Autodesk Inventor part; units mm, degrees
ref_plane "YZ Plane" through (0, 0, 0) normal (1, 0, 0) x (0, 1, 0)
ref_plane "XZ Plane" through (0, 0, 0) normal (0, 1, 0) x (-1, 0, 0)
ref_plane "XY Plane" through (0, 0, 0) normal (0, 0, 1) x (1, 0, 0)
sketch "Sketch1" plane through (0, 0, 0) normal (0, 1, 0) x (-1, 0, 0)
  circle A0 centre (0, 0) radius 3.9
  dimension "d0" = 7.8
extrude "Extrusion1" add sketch "Sketch1" along normal blind 5.2
sketch "Sketch2" plane through (0, 0, 0) normal (0, -1, 0) x (1, 0, 0)
  circle A0 centre (0, 0) radius 5.5
  dimension "d3" = 11
extrude "Extrusion2" add sketch "Sketch2" along normal blind 16.5
sketch "Sketch3" plane through (0, 5.2, 0) normal (0, 1, 0) x (1, 0, 0)
  circle A0 centre (0, 0) radius 2.9
  circle A1 centre (0, 0) radius 1
  dimension "d6" = 5.8
  dimension "d7" = 2
extrude "Extrusion3" cut sketch "Sketch3" against normal blind 10
fillet "Fillet1" radius 1 1 edges at (-1, 5.2, 0)
properties part number "Strom"
Part model, mm, in its own coordinate system. A direction names the side the tool comes from. Coordinates: 2 decimals unless noted, no trailing zeros. Order: outer loops, then holes, each group sorted by start corner. A loop starts at its lowest first (then second) coordinate and runs counter-clockwise, first axis right, second up. Notation, with made-up numbers: M 40.5,-17 L 67.5,-17 A6 cw 67.5,-11 Z; hole C 43,-31 d3. An arc over 180 degrees is marked long. One line per question, with ' | ' between items.
Q1. Drill centre lines: line 1 (Z direction, x = 0, y = 2); line 2 (Z direction, x = 0, y = -2); line 3 (X direction, y = 2.5, z = -0.5). Where is each one in solid material? Low to high.
A:
line 1: z = -3.9 to -2.9, -1 to 1, 2.9 to 3.9 | line 2: z = -5.5 to -2.9, -1 to 1, 2.9 to 5.5 | line 3: x = -3.87 to -2.86, -0.87 to 0.87, 2.86 to 3.87
Q2. Slice it at D-D (y = -7.25). Give the cut face in (x, z).
A:
outline: C 0,0 d11
Q3. Slice it at A-A (z = 0). Give the cut face in (x, y), and give its area (3 significant figures).
A:
outline: M -5.5,-16.5 L 5.5,-16.5 L 5.5,0 L 3.9,0 L 3.9,5.2 L 2.9,5.2 L 2.9,-4.8 L 1,-4.8 L 1,4.2 A1 ccw -1,4.2 L -1,-4.8 L -2.9,-4.8 L -2.9,5.2 L -3.9,5.2 L -3.9,0 L -5.5,0 Z | area: 184 mm^2
Q4. Slice it at C-C (y = -2.5). Give the cut face in (x, z), and give its area (3 significant figures).
A:
outline: C 0,0 d11; C 0,0 d2; hole C 0,0 d5.8 | area: 71.8 mm^2
Q5. 3-axis set-ups, long thin cutter, end or side, ignore diameter. For faces 1 (the face through (1, 5.2, 3)), 2 (the face through (2.87, 2.56, -2.64)): which of +Z, -Z, +X, -X, +Y, -Y reach the whole face in a straight line?
A:
face 1: +Z, -Z, +X, -X, +Y | face 2: +Y
Q6. Pin check, flat tips, straight feed: P1, Ø4.5, axis at x = 0.5, z = 0, coming from the +Y side; P2, Ø1, axis at x = 4, z = -4, coming from the +Y side; P3, Ø1, axis at x = -3, y = -13.5, coming from the -Z side; P4, Ø4, axis at y = -4, z = 2.5, coming from the -X side. Stop position of each tip, or through.
A:
P1: stops at y = 5.2 | P2: stops at y = 0 | P3: stops at z = -4.9 | P4: stops at x = -5.48
Q7. Slice it at B-B (x = 0). Give the cut face in (y, z).
A:
outline: M -16.5,-5.5 L 0,-5.5 L 0,-3.9 L 5.2,-3.9 L 5.2,-2.9 L -4.8,-2.9 L -4.8,-1 L 4.2,-1 A1 ccw 4.2,1 L -4.8,1 L -4.8,2.9 L 5.2,2.9 L 5.2,3.9 L 0,3.9 L 0,5.5 L -16.5,5.5 Z
